Part model, mm, in its own coordinate system. A direction names the side the tool comes from. Round coordinates to 2 decimals unless told otherwise and drop trailing zeros. Write each loop counter-clockwise with the first axis right and the second up, starting at its lowest first coordinate (ties: lowest second). Pieces come first, ordered by that corner, then holes. Notation, with made-up numbers: (5.25, 56) -> (16.25, 56) arc R27 ccw to (16.25, 95) -> close; hole circle Ø3 at (-8.5, 39.25). An arc over 180 degrees is marked (long way). Return JSON: item names as keys, results as strings. Group by question number.
```python
from build123d import *

# Parameters (mm, degrees)
F1_DEPTH    = 25
F2_T1_DEPTH = 25
F2_T3_DEPTH = 33.2865856195
F2_T5_DEPTH = 35.1375068729
F2_T7_DEPTH = 26.2439265081
F2_T9_DEPTH = 29.0269565503
F3_T1_DEPTH = 64.9996021944
F3_T3_DEPTH = 54.4201853444
F3_T5_DEPTH = 62.5652900515
F3_T7_DEPTH = 70.9771112235
F4_R        = 14.1322148091
F5_DEPTH    = 3
F6_R        = 2


# Not quite as in the source:
# - a fillet or chamfer that OpenCascade refuses, or shapes differently, is made with other operations: its cross-section is extruded or revolved along the edge and cut away or added


with BuildPart() as f1:
    # F0 (on Front) → F1 (new body)
    with BuildSketch(Plane.XZ):
        with BuildLine():
            Line((-81.2098225326, -15.6771827859), (-68.6711987798, -15.6771827859))
            ThreePointArc((-68.6711987798, -15.6771827859), (-57.1419560716, -20.274533801), (-46.4318082669, -14.0014318744))
            Line((-46.4318082669, -14.0014318744), (33.4813362922, -14.0014318744))
            ThreePointArc((33.4813362922, -14.0014318744), (48.0187694937, -21.717844135), (60.0034566781, -10.4374516171))
            Line((60.0034566781, -10.4374516171), (71.1715072393, -9.4995843247))
            Line((71.1715072393, -9.4995843247), (71.1715072393, 10.7058854774))
            Line((71.1715072393, 10.7058854774), (29.5542683452, 22.7688532323))
            Line((29.5542683452, 22.7688532323), (0, 25.1814462245))
            Line((0, 25.1814462245), (-33.7763093412, 13.7216281146))
            Line((-33.7763093412, 13.7216281146), (-66.3463175297, 13.7216281146))
            Line((-66.3463175297, 13.7216281146), (-73.5840946436, 9.8011633381))
            Line((-73.5840946436, 9.8011633381), (-89.2659574747, 0))
            Line((-89.2659574747, 0), (-87.1549323201, -4.9759717658))
            Line((-87.1549323201, -4.9759717658), (-81.2098225326, -15.6771827859))
        make_face()
    extrude(amount=F1_DEPTH)

    # F2: fillet of radius 8 on 5 edges, made by hand

    # F2_s2 → F2_t1 (join)
    with BuildSketch(Plane.XZ):
        with BuildLine():
            ThreePointArc((-32.5261230106, 14.1457984349), (-33.7939263524, 13.8283829823), (-35.0964935411, 13.7216281146))
            Line((-35.0964935411, 13.7216281146), (-33.7763093412, 13.7216281146))
            Line((-33.7763093412, 13.7216281146), (-32.5261230106, 14.1457984349))
        make_face()
    extrude(amount=F2_T1_DEPTH)

    # F2_s4 → F2_t3 (cut)
    with BuildSketch(Plane.XZ.offset(-4.1432928098)):
        with BuildLine():
            ThreePointArc((1.6518224825, 25.0466035919), (0.0208109602, 25.012860503), (-1.569444032, 24.6489563376))
            Line((-1.569444032, 24.6489563376), (0, 25.1814462245))
            Line((0, 25.1814462245), (1.6518224825, 25.0466035919))
        make_face()
    extrude(amount=F2_T3_DEPTH, mode=Mode.SUBTRACT)

    # F2_s6 → F2_t5 (cut)
    with BuildSketch(Plane.XZ.offset(-5.0687534365)):
        with BuildLine():
            ThreePointArc((-64.3188161551, 13.7216281146), (-66.284181416, 13.4764549593), (-68.1290829763, 12.7559629624))
            Line((-68.1290829763, 12.7559629624), (-66.3463175297, 13.7216281146))
            Line((-66.3463175297, 13.7216281146), (-64.3188161551, 13.7216281146))
        make_face()
    extrude(amount=F2_T5_DEPTH, mode=Mode.SUBTRACT)

    # F2_s8 → F2_t7 (cut)
    with BuildSketch(Plane.XZ.offset(-0.6219632541)):
        with BuildLine():
            ThreePointArc((-73.365339754, 9.9196556357), (-73.5821478307, 9.7978216209), (-73.7950641631, 9.669307401))
            Line((-73.7950641631, 9.669307401), (-73.5840946436, 9.8011633381))
            Line((-73.5840946436, 9.8011633381), (-73.365339754, 9.9196556357))
        make_face()
    extrude(amount=F2_T7_DEPTH, mode=Mode.SUBTRACT)

    # F2_s10 → F2_t9 (cut)
    with BuildSketch(Plane.XZ.offset(-2.0134782752)):
        with BuildLine():
            ThreePointArc((30.3278196103, 22.544635475), (29.5469574945, 22.7290808385), (28.751547216, 22.8343814784))
            Line((28.751547216, 22.8343814784), (29.5542683452, 22.7688532323))
            Line((29.5542683452, 22.7688532323), (30.3278196103, 22.544635475))
        make_face()
    extrude(amount=F2_T9_DEPTH, mode=Mode.SUBTRACT)

    # F3: fillet of radius 10 on 4 edges, made by hand

    # F3_s2 → F3_t1 (cut)
    with BuildSketch(Plane.XZ.offset(-19.9998010972)):
        with BuildLine():
            ThreePointArc((-87.1549323201, -4.9759717658), (-86.1010433194, 0.2823042988), (-82.4820383293, 4.239949063))
            Line((-82.4820383293, 4.239949063), (-89.2659574747, 0))
            Line((-89.2659574747, 0), (-87.1549323201, -4.9759717658))
        make_face()
    extrude(amount=F3_T1_DEPTH, mode=Mode.SUBTRACT)

    # F3_s4 → F3_t3 (cut)
    with BuildSketch(Plane.XZ.offset(-14.7100926722)):
        with BuildLine():
            ThreePointArc((-75.3257854638, -15.6771827859), (-80.3970650538, -14.2958905382), (-84.0673608071, -10.5336074498))
            Line((-84.0673608071, -10.5336074498), (-81.2098225326, -15.6771827859))
            Line((-81.2098225326, -15.6771827859), (-75.3257854638, -15.6771827859))
        make_face()
    extrude(amount=F3_T3_DEPTH, mode=Mode.SUBTRACT)

    # F3_s6 → F3_t5 (cut)
    with BuildSketch(Plane.XZ.offset(-18.7826450258)):
        with BuildLine():
            ThreePointArc((63.9554677121, 12.7974911304), (69.1664933159, 9.1995068855), (71.1715072393, 3.1928274671))
            Line((71.1715072393, 3.1928274671), (71.1715072393, 10.7058854774))
            Line((71.1715072393, 10.7058854774), (63.9554677121, 12.7974911304))
        make_face()
    extrude(amount=F3_T5_DEPTH, mode=Mode.SUBTRACT)

    # F3_s8 → F3_t7 (cut)
    with BuildSketch(Plane.XZ.offset(-22.9885556118)):
        with BuildLine():
            ThreePointArc((71.1715072393, -0.30416208), (68.532496131, -7.0729021797), (62.0083387319, -10.2690862168))
            Line((62.0083387319, -10.2690862168), (71.1715072393, -9.4995843247))
            Line((71.1715072393, -9.4995843247), (71.1715072393, -0.30416208))
        make_face()
    extrude(amount=F3_T7_DEPTH, mode=Mode.SUBTRACT)

    # F4 (on face) → F5 (cut)
    with BuildSketch(Plane.XZ.offset(25)):
        Polygon((0.0208109602, 22.1540294588), (-19.880797714, 14.1719523817), (23.1445431709, 15.3400599957), (26.0648149997, 20.0124960393), align=None)
        with Locations((-58.2038164139, -6.1822682619)):
            Circle(F4_R)
        with Locations((46.1366328286, -7.7115220987)):
            Circle(F4_R)
    extrude(amount=-F5_DEPTH, mode=Mode.SUBTRACT)

    # F6
    f6_edges = [f1.edges().sort_by_distance(p)[0] for p in [
        (-71.998492, -25, -15.677183),
        (-86.101043, -25, 0.282304),
        (-78.138551, -25, 6.954628),
        (-6.475236, -25, -14.001432),
        (-80.397065, -25, -14.295891),
        (-85.611147, -25, -7.75479),
        (-73.582148, -25, 9.797822),
        (-70.747211, -25, 11.337809),
        (-66.284181, -25, 13.476455),
        (-49.707655, -25, 13.721628),
        (-33.793926, -25, 13.828383),
        (-17.047784, -25, 19.397377),
        (0.020811, -25, 25.012861),
        (15.201685, -25, 23.940493),
        (29.546957, -25, 22.729081),
        (47.141644, -25, 17.671063),
        (69.166493, -25, 9.199507),
        (71.171507, -25, 1.444333),
        (68.532496, -25, -7.072902),
        (61.005898, -25, -10.353269),
    ]]
    fillet(f6_edges, radius=F6_R)

    # F7: F1 across plane


with BuildPart() as f1_1:
    add(f1.part)
    add(f1.part.mirror(Plane.XZ))


solid = f1_1.part
```
Item 1: Flat gauge pins, fed straight in: P1, Ø17, axis at x = -58.2, z = -6.18, coming from the +Y side; P2, Ø8, axis at y = 11.5, z = -16.5, coming from the +X side; P3, Ø23.5, axis at x = -45, y = 4.5, coming from the +Z side. Where does each tip first touch, or does it go through?
Item 2: Two-plate mould, pull along X, no slides. Class faces 4 (the face through (-72, 0, -15.677)), 5 (the face through (-16.64, 24.43, 18.9)), 6 (the face through (46, -22, -8)): released by +X, released by -X, zero draft, split by the parting line, or undercut.
Item 3: Cut at B-B (y = -16). Write the cut outline in (x, z).
Item 4: Wall check: L1, parallel to Y at x = -7, z = 15; L2, parallel to Z at x = -40.5, y = 6; L3, parallel to X at y = -16.5, z = 3. Give the ranges that are in metal, low to high.
Item 5: Cut at A-A (x = -38). Write the cut outline in (y, z).
Item 6: Which spindle directions (+Z, -Z, +X, -X, +Y, -Y) get a long thin tool onto all of the face, cutting with end or side? Do faces 1 (the face through (-58.825, -23.521, 7.936)), 2 (the face through (-58.825, 23.521, 7.936)), 3 (the face through (-85.1, 24.4, -7.5)). Say none if no direction does.
Checks:
{
 "1": {"P1": "stops at y = 22", "P2": "stops at x = 59.43", "P3": "stops at z = 13.94"},
 "2": {"face 4": "zero draft", "face 5": "released by -X", "face 6": "undercut"},
 "3": {"outline": "(-87.15, -4.98) -> (-84.07, -10.53) arc R10 ccw to (-75.33, -15.68) -> (-68.67, -15.68) arc R14.13 ccw to (-46.43, -14) -> (33.48, -14) arc R14.13 ccw to (60, -10.44) -> (62.01, -10.27) arc R10 ccw to (71.17, -0.3) -> (71.17, 3.19) arc R10 ccw to (63.96, 12.8) -> (30.33, 22.54) arc R8 ccw to (28.75, 22.83) -> (1.65, 25.05) arc R8 ccw to (-1.57, 24.65) -> (-32.53, 14.15) arc R8 cw to (-35.1, 13.72) -> (-64.32, 13.72) arc R8 ccw to (-68.13, 12.76) -> (-73.37, 9.92) arc R8 ccw to (-73.8, 9.67) -> (-82.48, 4.24) arc R10 ccw to start"},
 "4": {"L1": "y = -22 to 22", "L2": "z = -14 to 13.72", "L3": "x = -84.08 to 71.17"},
 "5": {"outline": "(-25, -12) arc R2 ccw to (-23, -14) -> (23, -14) arc R2 ccw to (25, -12) -> (25, 11.72) arc R2 ccw to (23, 13.72) -> (-23, 13.72) arc R2 ccw to (-25, 11.72) -> close"},
 "6": {"face 1": "-Y", "face 2": "+Y", "face 3": "-Z, -X, +Y"}
}
